from build123d import *

# Parameters (mm, degrees)
SKETCH1_R                       = 20
SKETCH1_R_2                     = 1
BOSS_EXTRUDE1_DEPTH             = 21.55
TAP_DRILL_FOR_M5X0_8_TAP1_D     = 4.2
TAP_DRILL_FOR_M5X0_8_TAP1_DEPTH = 5
TAP_DRILL_FOR_M5X0_8_TAP1_TIP   = 1.2618073
SKETCH4_W                       = 2.79
SKETCH4_H                       = 6.5
CUT_EXTRUDE1_DEPTH              = 19.05
CIRPATTERN1_COUNT               = 14
SKETCH5_R                       = 6
SKETCH5_R_2                     = 5
SKETCH5_R_3                     = 1
CUT_EXTRUDE2_DEPTH              = 1
CUT_EXTRUDE3_DEPTH              = 21.55
SKETCH7_R                       = 10.5
CUT_EXTRUDE4_DEPTH              = 6.55
FILLET4_R                       = 2
FILLET5_R                       = 4


with BuildPart() as part:
    # Sketch1 → Boss-Extrude1 (new body)
    with BuildSketch(Plane.XY):
        with Locations((-11.822558412, 14.529752947)):
            Circle(SKETCH1_R)
        with Locations((-11.822558412, 14.529752947)):
            Circle(SKETCH1_R_2, mode=Mode.SUBTRACT)
    extrude(amount=BOSS_EXTRUDE1_DEPTH)

    # Tap Drill for M5x0.8 Tap1
    with Locations(Plane.XY.offset(21.55)):
        with Locations((-11.822558412, 14.529752947)):
            Hole(TAP_DRILL_FOR_M5X0_8_TAP1_D / 2, depth=TAP_DRILL_FOR_M5X0_8_TAP1_DEPTH)
            with Locations((0, 0, -(TAP_DRILL_FOR_M5X0_8_TAP1_DEPTH + TAP_DRILL_FOR_M5X0_8_TAP1_TIP / 2))):  # 118° drill point
                Cone(0, TAP_DRILL_FOR_M5X0_8_TAP1_D / 2, TAP_DRILL_FOR_M5X0_8_TAP1_TIP, mode=Mode.SUBTRACT)

    # Sketch4 → Cut-Extrude1 (cut)
    with BuildSketch(Plane.XY.offset(21.55)):
        with Locations((4.782441588, 14.529752947)):
            Rectangle(SKETCH4_W, SKETCH4_H)
    cut_extrude1 = extrude(amount=-CUT_EXTRUDE1_DEPTH, mode=Mode.SUBTRACT)

    # CirPattern1: Cut-Extrude1 ×14 about axis
    cirpattern1_axis = Axis((-11.822558412, 14.529752947, 0), (0, 0, 1))
    for i in range(1, CIRPATTERN1_COUNT):
        add(cut_extrude1.rotate(cirpattern1_axis, i * 360 / CIRPATTERN1_COUNT), mode=Mode.SUBTRACT)

    # Sketch5 → Cut-Extrude2 (cut)
    # profile 1 of 2: a face of its own
    with BuildSketch(Plane(origin=(0, 0, 0), x_dir=(-1, 0, 0), z_dir=(0, 0, -1))):
        with Locations((11.822558412, 14.529752947)):
            Circle(SKETCH5_R)
        with Locations((11.822558412, 14.529752947)):
            Circle(SKETCH5_R_2, mode=Mode.SUBTRACT)
    # profile 2 of 2: a face of its own
    with BuildSketch(Plane(origin=(0, 0, 0), x_dir=(-1, 0, 0), z_dir=(0, 0, -1))):
        with Locations((11.822558412, 14.529752947)):
            Circle(SKETCH5_R_2)
        with Locations((11.822558412, 14.529752947)):
            Circle(SKETCH5_R_3, mode=Mode.SUBTRACT)
    extrude(amount=-CUT_EXTRUDE2_DEPTH, mode=Mode.SUBTRACT)

    # Sketch6 → Cut-Extrude3 (cut)
    with BuildSketch(Plane.XY.offset(21.55)):
        Polygon((-16.822558412, 17.416002947), (-11.822558412, 20.295742519), (-6.822558412, 17.416002947), (-6.822558412, 11.643502947), (-11.822558412, 8.763763375), (-16.822558412, 11.643502947), align=None)
    extrude(amount=-CUT_EXTRUDE3_DEPTH, mode=Mode.SUBTRACT)

    # Sketch7 → Cut-Extrude4 (cut)
    with BuildSketch(Plane.XY.offset(21.55)):
        with Locations((-11.822558412, 14.529752947)):
            Circle(SKETCH7_R)
    extrude(amount=-CUT_EXTRUDE4_DEPTH, mode=Mode.SUBTRACT)

    # Fillet4
    fillet4_edges = [part.edges().sort_by_distance(p)[0] for p in [
        (-22.322558412, 14.529752947, 21.55),
    ]]
    fillet(fillet4_edges, radius=FILLET4_R)

    # Fillet5
    fillet5_edges = [part.edges().sort_by_distance(p)[0] for p in [
        (-22.322558412, 14.529752947, 15),
    ]]
    fillet(fillet5_edges, radius=FILLET5_R)


solid = part.part
Design review of the part built by this model. Coordinates are the model's own, in mm. A direction names the side the tool comes from. Coordinates: 2 decimals unless noted, no trailing zeros.
Item 1: For line 1 (Y direction, x = -14, z = 5); line 2 (Y direction, x = -15.5, z = 12); line 3 (Y direction, x = -21, z = 9.5), list the stretches that pass through material, from the lowest coordinate up.
Item 2: For pin 1 Ø4 at (x, z) = (-5.5, 3.5) entering from +Y; pin 2 Ø1 at (x, z) = (-26, 15.5) entering from +Y; pin 3 Ø3 at (x, z) = (4, 14.5) entering from +Y, all flat-tipped, find the tip position at first contact; note any pin that passes through.
Item 3: For faces 1 (the flat face through (-2.375, 2.61, 12.158)), 2 (the flat face through (-14.288, 10.183, 8.098)), list the 3-axis set-ups (+Z, -Z, +X, -X, +Y, -Y) from which the entire face can be reached by the end or side of a thin tool; tool diameter is ignored.
Item 4: The part is to be moulded in two halves that separate along X. For faces 3 (the flat face through (-9.288, 10.224, 8.098)), 4 (the flat face through (-28, 14, 2.5)), say which applies: pulls with the +X half, pulls with the -X half, needs draft (parallel to the pull), parting line crosses it, or undercut.
Item 5: Take a section at A-A, the plane z = 20.5. Count the separate pieces of the cut face and the enclosed holes in it, then the cut area to 3 significant figures.
The answers:
1. line 1: y = -5.35 to -3.44, -0.57 to 10.02, 19.04 to 29.63, 32.5 to 34.41
1. line 2: y = -5.13 to -3.09, -0.23 to 10.88, 18.18 to 29.29, 32.15 to 34.19
1. line 3: y = -3.24 to -1.17, 2.39 to 26.67, 30.23 to 32.3
2. pin 1: stops at y = 34.06
2. pin 2: stops at y = 29.12
2. pin 3: stops at y = 28.49
3. face 1: +Z
3. face 2: +Z, -Z
4. face 3: undercut
4. face 4: undercut
5. separate pieces: 1
5. enclosed holes: 15
5. area: 640 mm2
